Can you work these out from the drawing? Everything is in mm from the part's minimum corner. A direction names the side the tool comes from. Give positions to 0.01 mm unless a question says otherwise; leave off trailing zeros. Write each loop counter-clockwise with the first axis right and the second up, starting at its lowest first coordinate (ties: lowest second). Pieces come first, ordered by that corner, then holes. Notation, with made-up numbers: (27, 13.5) - (67, 13.5) arc R25 cw to (67, 32.5) - close; hole circle Ø1 at (23, -21). An arc over 180 degrees is marked (long way). Write each question's results on one line, items separated by ' | '. Start each with the question number.
Item 1: Will these pins go through, and if not, where does the flat tip stop? P1, Ø5, axis at x = 4.5, y = 10.5, coming from the -Z side; P2, Ø1.9, axis at x = 6.5, z = 2, coming from the -Y side.
Item 2: Which directions (+Z, -Z, +X, -X, +Y, -Y) give clear straight access to the entire face, cutting with the end or side of a thin tool? Please do the marked faces 1 and 2.
Item 3: Suppose I cut it at B-B on z = 0.75. List the corners of the cut face in (x, y) for me.
Item 4: Suppose I cut it at C-C on x = 7.75. List the corners of the cut face in (y, z) for me, then the cut area to 3 significant figures.
Item 5: Suppose I cut it at A-A on y = 6. List the corners of the cut face in (x, z) for me.
Item 6: We'd pull the mould along X, two halves only. Please class the marked faces 3, 4 and 5: +X half, -X half, draft (parallel to the pull), parting line (faces both ways), or undercut.
Item 7: Please list where these lines run through material, in increasing order: line 1 along X through (y, z) = (9.5, 3); line 2 along Y through (x, z) = (7.95, 3.15); line 3 along Y through (x, z) = (3.75, 4.75).
Item 8: Suppose I cut it at D-D on y = 10.74. List the corners of the cut face in (x, z) for me.
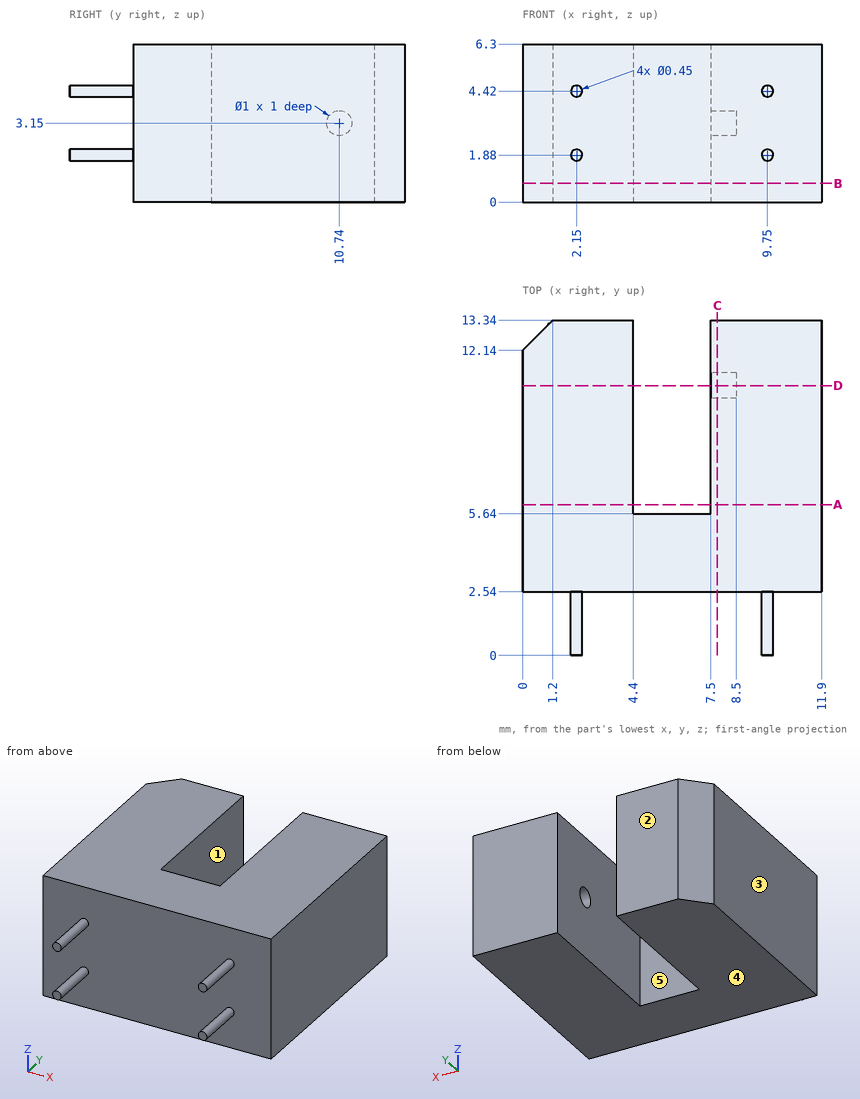
Checked values:
1) P1: stops at z = 0 | P2: stops at y = 2.54
2) face 1: +Z, -Z, +Y | face 2: +Z, -Z, +X, -X, +Y
3) outline: (0, 2.54) - (11.9, 2.54) - (11.9, 13.34) - (7.5, 13.34) - (7.5, 5.64) - (4.4, 5.64) - (4.4, 13.34) - (1.2, 13.34) - (0, 12.14) - close
4) outline: (2.54, 0) - (13.34, 0) - (13.34, 6.3) - (2.54, 6.3) - close; hole circle Ø1 at (10.74, 3.15) | area: 67.3 mm^2
5) outline: (0, 0) - (4.4, 0) - (4.4, 6.3) - (0, 6.3) - close; (7.5, 0) - (11.9, 0) - (11.9, 6.3) - (7.5, 6.3) - close
6) face 3: -X half | face 4: draft | face 5: undercut
7) line 1: x = 0 to 4.4, 7.5 to 11.9 | line 2: y = 2.54 to 10.24, 11.24 to 13.34 | line 3: y = 2.54 to 13.34
8) outline: (0, 0) - (4.4, 0) - (4.4, 6.3) - (0, 6.3) - close; (7.5, 0) - (11.9, 0) - (11.9, 6.3) - (7.5, 6.3) - (7.5, 3.65) - (8.5, 3.65) - (8.5, 2.65) - (7.5, 2.65) - close
